Could you check a few things on this model? Use its own coordinates, in mm. Face numbers are marked on the shaded views. Round coordinates to 2 decimals unless told otherwise and drop trailing zeros. Loops run counter-clockwise (first coordinate to the right, second up) from the corner with the lowest first, then second, coordinate; pieces in that order, holes last. Notation, with made-up numbers: (-40, 60) -> (-24, 60) arc R16 cw to (-24, 69) -> close; hole circle Ø3 at (71.5, 14). An arc over 180 degrees is marked (long way). One line per item, written item: value.
```python
from build123d import *

# Parameters (mm, degrees)
BOSS_EXTRUDE1_DEPTH = 8
BOSS_EXTRUDE2_START = 8
SKETCH3_7_W         = 139.5
SKETCH3_7_H         = 11.9
BOSS_EXTRUDE2_DEPTH = 15
FILLET1_R           = 8
CUT_EXTRUDE1_REACH  = 139.901
BOSS_EXTRUDE3_DEPTH = 12.5
CUT_EXTRUDE2_REACH  = 232.432
SKETCH6_R           = 1.375
BOSS_EXTRUDE4_DEPTH = 99.5
FILLET2_R           = 5
CUT_EXTRUDE3_REACH  = 140.357
SKETCH9_W           = 70
SKETCH9_H           = 11.9
CUT_EXTRUDE4_REACH  = 142.044
CUT_EXTRUDE5_REACH  = 142.044
SKETCH11_R          = 22


with BuildPart() as part:
    # Sketch3 → Boss-Extrude1 (new body)
    with BuildSketch(Plane(origin=(0, 0, 0), x_dir=(1, 0, 0), z_dir=(0, 1, 0))):
        with BuildLine():
            Line((-75, 110), (75, 110))
            ThreePointArc((75, 110), (78.535533906, 108.535533906), (80, 105))
            Line((80, 105), (80, -105))
            ThreePointArc((80, -105), (78.535533906, -108.535533906), (75, -110))
            Line((75, -110), (-75, -110))
            ThreePointArc((-75, -110), (-78.535533906, -108.535533906), (-80, -105))
            Line((-80, -105), (-80, 105))
            ThreePointArc((-80, 105), (-78.535533906, 108.535533906), (-75, 110))
        make_face()
    extrude(amount=BOSS_EXTRUDE1_DEPTH)

    # Sketch3<7> → Boss-Extrude2 (add)
    with BuildSketch(Plane(origin=(0, 0, 0), x_dir=(1, 0, 0), z_dir=(0, 1, 0)).offset(BOSS_EXTRUDE2_START)):
        with Locations((0, 98.95)):
            Rectangle(SKETCH3_7_W, SKETCH3_7_H)
    extrude(amount=BOSS_EXTRUDE2_DEPTH)

    # Fillet1
    # the kernel refuses this fillet: 8 mm, written as the material it takes off along each edge
    with BuildSketch(Plane(origin=(89.75, 23, -93), x_dir=(0, -1, 0), z_dir=(-1, 0, 0)), Plane(origin=(-89.75, 23, -104.9), x_dir=(0, -1, 0), z_dir=(1, 0, 0))) as fillet1_piece_1:
        with BuildLine():
            CenterArc((FILLET1_R, -FILLET1_R), FILLET1_R, 90, 90)
            Line((0, -FILLET1_R), (0, 0))
            Line((0, 0), (FILLET1_R, 0))
        make_face()
    extrude(amount=179.5, mode=Mode.SUBTRACT)

    # Sketch4 → Cut-Extrude1 (cut, up to next)
    with BuildSketch(Plane.XZ, mode=Mode.PRIVATE) as cut_extrude1_sk1:
        with BuildLine():
            Line((-55, 0), (55, 0))
            ThreePointArc((55, 0), (58.535533906, -1.464466094), (60, -5))
            Line((60, -5), (60, -35))
            ThreePointArc((60, -35), (58.535533906, -38.535533906), (55, -40))
            Line((55, -40), (-55, -40))
            ThreePointArc((-55, -40), (-58.535533906, -38.535533906), (-60, -35))
            Line((-60, -35), (-60, -5))
            ThreePointArc((-60, -5), (-58.535533906, -1.464466094), (-55, 0))
        make_face()
    cut_extrude1_tool1 = extrude(cut_extrude1_sk1.sketch, amount=-CUT_EXTRUDE1_REACH, mode=Mode.PRIVATE) & part.part
    add(cut_extrude1_tool1.solids().sort_by_distance((0, 0, -20))[0], mode=Mode.SUBTRACT)

    # Sketch5 → Boss-Extrude3 (add)
    with BuildSketch(Plane(origin=(0, 8, 0), x_dir=(1, 0, 0), z_dir=(0, 1, 0))):
        with BuildLine():
            ThreePointArc((-69.5, -104.5), (-73.035533906, -103.035533906), (-74.5, -99.5))
            Line((-74.5, -99.5), (-74.5, 29.5))
            ThreePointArc((-74.5, 29.5), (-73.035533906, 33.035533906), (-69.5, 34.5))
            Line((-69.5, 34.5), (-69.5, -99.5))
            Line((-69.5, -99.5), (69.5, -99.5))
            Line((69.5, -99.5), (69.5, 34.5))
            ThreePointArc((69.5, 34.5), (73.035533906, 33.035533906), (74.5, 29.5))
            Line((74.5, 29.5), (74.5, -99.5))
            ThreePointArc((74.5, -99.5), (73.035533906, -103.035533906), (69.5, -104.5))
            Line((69.5, -104.5), (-69.5, -104.5))
        make_face()
    extrude(amount=BOSS_EXTRUDE3_DEPTH)

    # Sketch6 → Cut-Extrude2 (cut, up to next)
    with BuildSketch(Plane(origin=(0, 0, -104.9), x_dir=(-1, 0, 0), z_dir=(0, 0, -1)), mode=Mode.PRIVATE) as cut_extrude2_sk1:
        with Locations((-64.75, 11.5)):
            Circle(SKETCH6_R)
    cut_extrude2_tool1 = extrude(cut_extrude2_sk1.sketch, amount=-CUT_EXTRUDE2_REACH, mode=Mode.PRIVATE) & part.part
    # Sketch6 → Cut-Extrude2 (cut, up to next)
    with BuildSketch(Plane(origin=(0, 0, -104.9), x_dir=(-1, 0, 0), z_dir=(0, 0, -1)), mode=Mode.PRIVATE) as cut_extrude2_sk2:
        with Locations(Location((64.75, 11.5, 0), (0, 0, 180))):
            Circle(SKETCH6_R)
    cut_extrude2_tool2 = extrude(cut_extrude2_sk2.sketch, amount=-CUT_EXTRUDE2_REACH, mode=Mode.PRIVATE) & part.part
    add(cut_extrude2_tool1.solids().sort_by_distance((64.75, 11.5, -104.9))[0], mode=Mode.SUBTRACT)
    add(cut_extrude2_tool2.solids().sort_by_distance((-64.75, 11.5, -104.9))[0], mode=Mode.SUBTRACT)

    # Sketch8 → Boss-Extrude4 (add)
    with BuildSketch(Plane(origin=(0, 0, 99.5), x_dir=(-1, 0, 0), z_dir=(0, 0, -1))):
        with BuildLine():
            Line((-38.026756028, 8), (-31.313789331, 8))
            ThreePointArc((-31.313789331, 8), (-40.187326194, 20.238486432), (-28.95, 30.35))
            Line((-28.95, 30.35), (28.95, 30.35))
            ThreePointArc((28.95, 30.35), (40.187326194, 20.238486432), (31.313789331, 8))
            Line((31.313789331, 8), (38.026756028, 8))
            ThreePointArc((38.026756028, 8), (42.413004865, 23.870529017), (28.95, 33.35))
            Line((28.95, 33.35), (-28.95, 33.35))
            ThreePointArc((-28.95, 33.35), (-42.413004865, 23.870529017), (-38.026756028, 8))
        make_face()
    extrude(amount=BOSS_EXTRUDE4_DEPTH)

    # Fillet2
    fillet2_edges = [part.edges().sort_by_distance(p)[0] for p in [
        (-38.026756028, 8, 49.75),
        (38.026756028, 8, 49.75),
    ]]
    fillet(fillet2_edges, radius=FILLET2_R)

    # Sketch9 → Cut-Extrude3 (cut, up to next)
    with BuildSketch(Plane(origin=(0, 8, 0), x_dir=(1, 0, 0), z_dir=(0, 1, 0)), mode=Mode.PRIVATE) as cut_extrude3_sk1:
        with Locations((0, 98.95)):
            Rectangle(SKETCH9_W, SKETCH9_H)
    cut_extrude3_tool1 = extrude(cut_extrude3_sk1.sketch, amount=CUT_EXTRUDE3_REACH, mode=Mode.PRIVATE) & part.part
    add(cut_extrude3_tool1.solids().sort_by_distance((0, 8, -98.95))[0], mode=Mode.SUBTRACT)

    # Sketch10 → Cut-Extrude4 (cut, up to next)
    with BuildSketch(Plane(origin=(0, 33.35, 0), x_dir=(1, 0, 0), z_dir=(0, 1, 0)), mode=Mode.PRIVATE) as cut_extrude4_sk1:
        Polygon((4.409098458, -49.75), (20.95, -85.422252035), (20.95, -14.077747965), align=None)
    cut_extrude4_tool1 = extrude(cut_extrude4_sk1.sketch, amount=-CUT_EXTRUDE4_REACH, mode=Mode.PRIVATE) & part.part
    # Sketch10 → Cut-Extrude4 (cut, up to next)
    with BuildSketch(Plane(origin=(0, 33.35, 0), x_dir=(1, 0, 0), z_dir=(0, 1, 0)), mode=Mode.PRIVATE) as cut_extrude4_sk2:
        Polygon((0, -59.258700058), (-14.95, -91.5), (14.95, -91.5), align=None)
    cut_extrude4_tool2 = extrude(cut_extrude4_sk2.sketch, amount=-CUT_EXTRUDE4_REACH, mode=Mode.PRIVATE) & part.part
    # Sketch10 → Cut-Extrude4 (cut, up to next)
    with BuildSketch(Plane(origin=(0, 33.35, 0), x_dir=(1, 0, 0), z_dir=(0, 1, 0)), mode=Mode.PRIVATE) as cut_extrude4_sk3:
        Polygon((14.95, -8), (-14.95, -8), (0, -40.241299942), align=None)
    cut_extrude4_tool3 = extrude(cut_extrude4_sk3.sketch, amount=-CUT_EXTRUDE4_REACH, mode=Mode.PRIVATE) & part.part
    # Sketch10 → Cut-Extrude4 (cut, up to next)
    with BuildSketch(Plane(origin=(0, 33.35, 0), x_dir=(1, 0, 0), z_dir=(0, 1, 0)), mode=Mode.PRIVATE) as cut_extrude4_sk4:
        Polygon((-20.95, -14.077747965), (-20.95, -85.422252035), (-4.409098458, -49.75), align=None)
    cut_extrude4_tool4 = extrude(cut_extrude4_sk4.sketch, amount=-CUT_EXTRUDE4_REACH, mode=Mode.PRIVATE) & part.part
    add(cut_extrude4_tool1.solids().sort_by_distance((15.436366, 33.35, 49.75))[0], mode=Mode.SUBTRACT)
    add(cut_extrude4_tool2.solids().sort_by_distance((0, 33.35, 80.7529))[0], mode=Mode.SUBTRACT)
    add(cut_extrude4_tool3.solids().sort_by_distance((0, 33.35, 18.7471))[0], mode=Mode.SUBTRACT)
    add(cut_extrude4_tool4.solids().sort_by_distance((-15.436366, 33.35, 49.75))[0], mode=Mode.SUBTRACT)

    # Sketch11 → Cut-Extrude5 (cut, up to next)
    with BuildSketch(Plane.XZ, mode=Mode.PRIVATE) as cut_extrude5_sk1:
        with Locations(Location((0, -64.78, 0), (0, 0, 270))):
            Circle(SKETCH11_R)
    cut_extrude5_tool1 = extrude(cut_extrude5_sk1.sketch, amount=-CUT_EXTRUDE5_REACH, mode=Mode.PRIVATE) & part.part
    add(cut_extrude5_tool1.solids().sort_by_distance((0, 0, -64.78))[0], mode=Mode.SUBTRACT)


solid = part.part
```
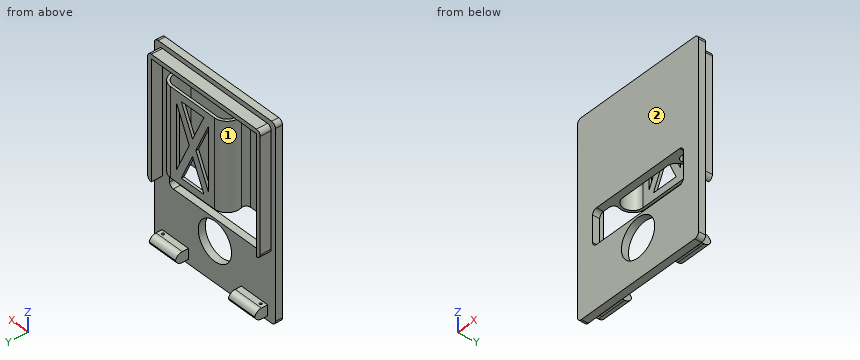
Item 1: If we section it at D-D on z = -90: List the corners of the cut face in (x, y) for me, plus the area to 3 significant figures.
Output:
outline: (-80, 0) -> (80, 0) -> (80, 8) -> (-80, 8) -> close
area: 1,280 mm²
Item 2: If we section it at A-A on x = 50: List the corners of the cut face in (y, z) for me.
Output:
outline: (0, -110) -> (8, -110) -> (8, -104.9) -> (15, -104.9) arc R8 ccw to (22.73, -98.95) arc R8 ccw to (15, -93) -> (8, -93) -> (8, -40) -> (0, -40) -> close; (0, 0) -> (8, 0) -> (8, 99.5) -> (20.5, 99.5) -> (20.5, 104.5) -> (8, 104.5) -> (8, 110) -> (0, 110) -> close
Item 3: I need wall thicknesses on line 1 (Z direction, x = -0.5, y = 5); line 2 (X direction, y = 30.5, z = 68); line 3 (Z direction, x = -14, y = 2). Which ranges of each line are inside material? Lowest first, please. Write a range as from..to.
Output:
line 1: z = -110..-86.77, -42.79..-40, 0..110
line 2: x = -37.52..-20.95, -12.87..-4.05, 4.05..12.87, 20.95..37.52
line 3: z = -110..-81.75, -47.81..-40, 0..110
Item 4: If we mould it in two halves opening along X, with no side actions, what happens to the marked faces 1 and 2? For each: released by +X, released by -X, zero draft, split by the parting line, or undercut.
Output:
face 1: undercut
face 2: zero draft
Item 5: If we section it at C-C on x = -8: Count the separate pieces of the cut face and the enclosed holes in it, plus the area to 3 significant figures.
Output:
separate pieces: 7
enclosed holes: 0
area: 1,340 mm²
Item 6: Will these pins go through, and if not, where does the flat tip stop? pin 1 Ø6 at (y, z) = (17.5, -99.5) entering from -X; pin 2 Ø4 at (y, z) = (13, 43) entering from +X; pin 3 Ø2 at (x, y) = (64.75, 11.5) entering from +Z.
Output:
pin 1: stops at x = -69.75
pin 2: stops at x = 74.5
pin 3: stops at z = 104.5
Item 7: If we section it at B-B on y = 3.5: List the corners of the cut face in (x, z) for me, plus the area to 3 significant figures.
Output:
outline: (-80, -105) arc R5 ccw to (-75, -110) -> (75, -110) arc R5 ccw to (80, -105) -> (80, 105) arc R5 ccw to (75, 110) -> (-75, 110) arc R5 ccw to (-80, 105) -> close; hole (-60, -35) arc R5 ccw to (-55, -40) -> (55, -40) arc R5 ccw to (60, -35) -> (60, -5) arc R5 ccw to (55, 0) -> (-55, 0) arc R5 ccw to (-60, -5) -> close; hole circle Ø44 at (0, -64.78)
area: 28,900 mm²
